Check sheet for the modelled part. Datum: model origin and axes. Units: mm. A direction names the side the tool comes from. Give positions to 0.01 mm unless a question says otherwise; leave off trailing zeros. Loops run counter-clockwise (first coordinate to the right, second up) from the corner with the lowest first, then second, coordinate; pieces in that order, holes last. Notation, with made-up numbers: (-34.75, -27.5) -> (-18.75, -27.5) arc R31 cw to (-18.75, -0.5) -> close; hole circle Ø11 at (-15, -31.75). An arc over 180 degrees is marked (long way). Write each question's results on one line, items separated by ' | '. Start each with the question number.
Item 1: Access from +Z, -Z, +X, -X, +Y, -Y to the whole of each face (thin tool, end or side, straight path). Record for faces 1 (the face through (5, -1, 0)), 2 (the face through (-6.524, 2.852, 0.217)), 3 (the face through (-5, -2, 0)).
Item 2: Scan lines: line 1 along X through (y, z) = (2.25, 0.25); line 2 along Z through (x, y) = (7.5, 2.05); line 3 along Z through (x, y) = (-2, -0.5). Record each from-to range of solid material in increasing order.
Item 3: Gauge pin test, flat ends, axial feed: pin 1 Ø1 at (y, z) = (3, -3) entering from +X; pin 2 Ø3 at (y, z) = (0, 0) entering from -X; pin 3 Ø2.5 at (x, z) = (-7.5, 0) entering from +Y; pin 4 Ø3 at (x, y) = (-7, 2) entering from +Z. Record the tip position at first contact, or that the pin passes through.
Item 4: Cross-section at B-B on x = 7.5. Enter the section's corners in (y, z).
Item 5: Mould release check, pull along X, two halves, no side actions. Record for faces 4 (the face through (10, -2, 0)), 5 (the face through (8.1, 2.4, 0.8)), 6 (the face through (0, -1, 1)): pulls with the +X half, pulls with the -X half, needs draft (parallel to the pull), parting line crosses it, or undercut.
Item 6: Cross-section at C-C on x = -7.5. Enter the section's corners in (y, z).
Item 7: Cross-section at A-A on z = 0. Enter the section's corners in (x, y), then the cut area to 3 significant figures.
from build123d import *

# Parameters (mm, degrees)
BOSS_EXTRUDE1_DEPTH      = 10
BOSS_EXTRUDE1_DEPTH_BACK = 10
SKETCH1_R                = 4
SKETCH2_R                = 1
CUT_EXTRUDE1_DEPTH       = 10
SKETCH3_R                = 2
CUT_EXTRUDE2_DEPTH       = 10
CUT_EXTRUDE4_REACH       = 13.489
CUT_EXTRUDE4_END_RADIUS  = 4
SKETCH4_R                = 1
FILLET1_R                = 0.5


with BuildPart() as part:
    # Sketch1 → Boss-Extrude1 (new, two sides: drawn at the far end of the back side and taken through both)
    with BuildSketch(Plane(origin=(0, 0, 0), x_dir=(0, 0, -1), z_dir=(1, 0, 0)).offset(-BOSS_EXTRUDE1_DEPTH_BACK)):
        Circle(SKETCH1_R)
    extrude(amount=BOSS_EXTRUDE1_DEPTH + BOSS_EXTRUDE1_DEPTH_BACK)

    # Sketch2 → Cut-Extrude1 (cut)
    with BuildSketch(Plane(origin=(10, 0, 0), x_dir=(0, 0, -1), z_dir=(1, 0, 0))):
        Circle(SKETCH2_R)
    extrude(amount=-CUT_EXTRUDE1_DEPTH, mode=Mode.SUBTRACT)

    # Sketch3 → Cut-Extrude2 (cut)
    with BuildSketch(Plane.ZY.offset(10)):
        Circle(SKETCH3_R)
    extrude(amount=-CUT_EXTRUDE2_DEPTH, mode=Mode.SUBTRACT)

    # Cut-Extrude4: up to this cylinder (the profile starts inside it)
    cut_extrude4_end = Plane(origin=(0, 0, 0), z_dir=(1, 0, 0)) * Cylinder(CUT_EXTRUDE4_END_RADIUS, 50.978, mode=Mode.PRIVATE)
    # Sketch4 → Cut-Extrude4 (cut, up to the surface)
    with BuildSketch(Plane(origin=(0, 0, 0), x_dir=(1, 0, 0), z_dir=(0, 1, 0)), mode=Mode.PRIVATE) as cut_extrude4_sk1:
        with Locations(Location((-7.5, 0, 0), (0, 0, 90))):
            Circle(SKETCH4_R)
    cut_extrude4_tool1 = extrude(cut_extrude4_sk1.sketch, amount=CUT_EXTRUDE4_REACH, mode=Mode.PRIVATE) & cut_extrude4_end
    add(cut_extrude4_tool1.solids().sort_by_distance((-7.5, 0, 0))[0], mode=Mode.SUBTRACT)
    # Sketch4 → Cut-Extrude4 (cut, up to the surface)
    with BuildSketch(Plane(origin=(0, 0, 0), x_dir=(1, 0, 0), z_dir=(0, 1, 0)), mode=Mode.PRIVATE) as cut_extrude4_sk2:
        with Locations(Location((7.5, 0, 0), (0, 0, 90))):
            Circle(SKETCH4_R)
    cut_extrude4_tool2 = extrude(cut_extrude4_sk2.sketch, amount=CUT_EXTRUDE4_REACH, mode=Mode.PRIVATE) & cut_extrude4_end
    add(cut_extrude4_tool2.solids().sort_by_distance((7.5, 0, 0))[0], mode=Mode.SUBTRACT)

    # Fillet1
    fillet1_edges = [part.edges().sort_by_distance(p)[0] for p in [
        (-10, 0, -2),
        (-10, 0, 4),
        (10, 0, 4),
        (10, 0, 1),
    ]]
    fillet(fillet1_edges, radius=FILLET1_R)


solid = part.part
Answer sheet:
1) face 1: +X, -X | face 2: +Y | face 3: -X
2) line 1: x = -9.94 to -8.47, -6.53 to 6.53, 8.47 to 10 | line 2: z = -3.43 to -1, 1 to 3.43 | line 3: z = -3.97 to -1.94, 1.94 to 3.97
3) pin 1: stops at x = 9.94 | pin 2: stops at x = 0 | pin 3: stops at y = 4 | pin 4: stops at z = 3.97
4) outline: (0, -1) arc R1 cw to (0, 1) -> (3.87, 1) arc R4 ccw (long way) to (3.87, -1) -> close
5) face 4: pulls with the +X half | face 5: undercut | face 6: pulls with the -X half
6) outline: (1.73, -1) arc R2 cw (long way) to (1.73, 1) -> (3.87, 1) arc R4 ccw (long way) to (3.87, -1) -> close
7) outline: (-10, -3.5) arc R0.5 ccw to (-9.5, -4) -> (9.5, -4) arc R0.5 ccw to (10, -3.5) -> (10, -1.5) arc R0.5 ccw to (9.5, -1) -> (0, -1) -> (0, -2) -> (-9.5, -2) arc R0.5 ccw to (-10, -2.5) -> close; (-10, 2.5) arc R0.5 ccw to (-9.5, 2) -> (-8.5, 2) -> (-8.5, 4) -> (-9.5, 4) arc R0.5 ccw to (-10, 3.5) -> close; (-6.5, 2) -> (0, 2) -> (0, 1) -> (6.5, 1) -> (6.5, 4) -> (-6.5, 4) -> close; (8.5, 1) -> (9.5, 1) arc R0.5 ccw to (10, 1.5) -> (10, 3.5) arc R0.5 ccw to (9.5, 4) -> (8.5, 4) -> close | area: 89.6 mm²
